Input: part model. Units: mm. Frame: model coordinates. A direction names the side the tool comes from. Coordinates: 2 decimals unless noted, no trailing zeros. Write each loop counter-clockwise with the first axis right and the second up, starting at its lowest first coordinate (ties: lowest second). Pieces come first, ordered by that corner, then holes.
1) Line query: L1, parallel to Y at x = 23.5, z = 0.7; L2, parallel to X at y = 24.5, z = 0.25; L3, parallel to Z at x = 19, y = 19.5. Output: solid intervals per line, ascending.
2) Draft query along Y for faces 3 (the flat face through (6, 6, -1.2)), 4 (the cylindrical face through (7.4, 32.5, 0.6)). Return one class per face: pulls with the +Y half, pulls with the -Y half, needs draft (parallel to the pull), parting line crosses it, or undercut.
3) Section query C-C (y = 103.5). Output: boundary loops of the cut face in (x, z).
4) Section query D-D (x = 6). Output: boundary loops of the cut face in (y, z).
5) Section query B-B (x = 18.5). Output: boundary loops of the cut face in (y, z).
6) Section query A-A (z = -0.6). Output: boundary loops of the cut face in (x, y), then the cut area to 3 significant figures.
7) Pin query (flat end, axial travel): pin 1 Ø0.6 at (x, z) = (6, -0.5) entering from -Y; pin 2 Ø0.6 at (y, z) = (104.5, -1) entering from -X; pin 3 Ø0.6 at (x, z) = (33.5, -0.5) entering from +Y. Return the tip coordinate at first contact, or that it passes through.
8) Set-up query: faces 1 (the flat face through (17, 56, 1.2)), 2 (the cylindrical face through (7.6, 77.5, 0.6)). Return all of +Z, -Z, +X, -X, +Y, -Y with unobstructed straight access to the full face (end or side cutting, diameter ignored); none if empty.
Autodesk Inventor part; units mm, degrees
ref_plane "YZ Plane" through (0, 0, 0) normal (1, 0, 0) x (0, 1, 0)
ref_plane "XZ Plane" through (0, 0, 0) normal (0, 1, 0) x (-1, 0, 0)
ref_plane "XY Plane" through (0, 0, 0) normal (0, 0, 1) x (1, 0, 0)
sketch "Skizze1" plane through (0, 0, 0) normal (0, 0, 1) x (1, 0, 0)
  line L0 (0, 0) -> (35, 0)
  line L1 (35, 0) -> (35, 110)
  line L2 (35, 110) -> (0, 110)
  line L3 (0, 110) -> (0, 0)
  line L4 (14, 105) -> (24, 105)
  line L5 (24, 105) -> (24, 100) construction
  line L6 (24, 100) -> (14, 100)
  line L7 (14, 100) -> (14, 105) construction
  line L8 (14, 10) -> (24, 10)
  line L9 (24, 10) -> (24, 5) construction
  line L10 (24, 5) -> (14, 5)
  line L11 (14, 5) -> (14, 10) construction
  line L12 (5, 90) -> (10, 90) construction
  line L13 (10, 90) -> (10, 80)
  line L14 (10, 80) -> (5, 80) construction
  line L15 (5, 80) -> (5, 90)
  line L16 (5, 30) -> (10, 30) construction
  line L17 (10, 30) -> (10, 20)
  line L18 (10, 20) -> (5, 20) construction
  line L19 (5, 20) -> (5, 30)
  line L20 (28, 90) -> (33, 90) construction
  line L21 (33, 90) -> (33, 80)
  line L22 (33, 80) -> (28, 80) construction
  line L23 (28, 80) -> (28, 90)
  line L24 (28, 30) -> (33, 30) construction
  line L25 (33, 30) -> (33, 20)
  line L26 (33, 20) -> (28, 20) construction
  line L27 (28, 20) -> (28, 30)
  line L28 (10, 80) -> (10, 30) construction
  line L29 (0, 55) -> (35, 55) construction
  arc A0 (5, 80) -> (10, 80) centre (7.5, 80) ccw
  arc A1 (10, 90) -> (5, 90) centre (7.5, 90) ccw
  arc A2 (33, 90) -> (28, 90) centre (30.5, 90) ccw
  arc A3 (28, 80) -> (33, 80) centre (30.5, 80) ccw
  arc A4 (24, 5) -> (24, 10) centre (24, 7.5) ccw
  arc A5 (14, 10) -> (14, 5) centre (14, 7.5) ccw
  arc A6 (5, 20) -> (10, 20) centre (7.5, 20) ccw
  arc A7 (28, 20) -> (33, 20) centre (30.5, 20) ccw
  arc A8 (33, 30) -> (28, 30) centre (30.5, 30) ccw
  arc A9 (10, 30) -> (5, 30) centre (7.5, 30) ccw
  arc A10 (24, 100) -> (24, 105) centre (24, 102.5) ccw
  arc A11 (14, 105) -> (14, 100) centre (14, 102.5) ccw
  line L30 (19, 10) -> (19, 100) construction
  line L31 (10, 85) -> (28, 85) construction
  point P0 (10, 55)
  point P1 (19, 85)
  dimension "d0" = 35
  dimension "d1" = 110
  dimension "d4" = 10
  dimension "d5" = 10
  dimension "d6" = 10
  dimension "d7" = 5
  dimension "d8" = 5
  dimension "d9" = 5
  dimension "d10" = 5
  dimension "d11" = 5
  dimension "d12" = 2
  dimension "d13" = 5
  dimension "d14" = 50
  dimension "d15" = 5
extrude "Extrusion2" add sketch "Skizze1" along normal blind 1.2
sketch "Skizze2" plane through (0, 0, 0) normal (0, 0, -1) x (-1, 0, 0)
  arc A0 (-28, 30) -> (-33, 30) centre (-30.5, 30) ccw construction
  line L0 (-28, 30) -> (-28, 20) construction
  arc A1 (-33, 20) -> (-28, 20) centre (-30.5, 20) ccw construction
  line L1 (-33, 20) -> (-33, 30) construction
  arc A2 (-28, 90) -> (-33, 90) centre (-30.5, 90) ccw construction
  line L2 (-28, 90) -> (-28, 80) construction
  arc A3 (-33, 80) -> (-28, 80) centre (-30.5, 80) ccw construction
  line L3 (-33, 80) -> (-33, 90) construction
  arc A4 (-5, 30) -> (-10, 30) centre (-7.5, 30) ccw construction
  line L4 (-5, 30) -> (-5, 20) construction
  arc A5 (-10, 20) -> (-5, 20) centre (-7.5, 20) ccw construction
  line L5 (-10, 20) -> (-10, 30) construction
  arc A6 (-5, 90) -> (-10, 90) centre (-7.5, 90) ccw construction
  line L6 (-5, 90) -> (-5, 80) construction
  arc A7 (-10, 80) -> (-5, 80) centre (-7.5, 80) ccw construction
  line L7 (-10, 80) -> (-10, 90) construction
  arc A8 (-24, 10) -> (-24, 5) centre (-24, 7.5) ccw construction
  line L8 (-24, 10) -> (-14, 10) construction
  arc A9 (-14, 5) -> (-14, 10) centre (-14, 7.5) ccw construction
  line L9 (-14, 5) -> (-24, 5) construction
  arc A10 (-24, 105) -> (-24, 100) centre (-24, 102.5) ccw construction
  line L10 (-24, 105) -> (-14, 105) construction
  arc A11 (-14, 100) -> (-14, 105) centre (-14, 102.5) ccw construction
  line L11 (-14, 100) -> (-24, 100) construction
  line L12 (0, 0) -> (-35, 0) construction
  line L13 (0, 110) -> (0, 0) construction
  line L14 (-35, 110) -> (0, 110) construction
  line L15 (-35, 0) -> (-35, 110) construction
  line L16 (-35, 3) -> (-30, 3)
  line L17 (-30, 3) -> (-30, 8)
  line L18 (-30, 8) -> (-35, 8)
  line L19 (-35, 8) -> (-35, 3)
  line L20 (-3, 3) -> (-8, 3)
  line L21 (-8, 3) -> (-8, 8)
  line L22 (-8, 8) -> (-3, 8)
  line L23 (-3, 8) -> (-3, 3)
  line L24 (-3, 102) -> (-8, 102)
  line L25 (-8, 102) -> (-8, 107)
  line L26 (-8, 107) -> (-3, 107)
  line L27 (-3, 107) -> (-3, 102)
  line L28 (-30, 107) -> (-35, 107)
  line L29 (-35, 107) -> (-35, 102)
  line L30 (-35, 102) -> (-30, 102)
  line L31 (-30, 102) -> (-30, 107)
  dimension "d18" = 5
  dimension "d19" = 5
  dimension "d20" = 5
  dimension "d21" = 5
  dimension "d22" = 3
  dimension "d23" = 0
  dimension "d24" = 3
  dimension "d25" = 3
extrude "Extrusion3" add sketch "Skizze2" along normal blind 1.2
properties part number "bett_V3_teil2_deckplatte_real" material "Holz (Walnuss)"
Answer:
1. L1: y = 0 to 5, 10 to 100, 105 to 110
1. L2: x = 0 to 5, 10 to 28, 33 to 35
1. L3: z = 0 to 1.2
2. face 3: needs draft
2. face 4: undercut
3. outline: (0, 0) - (3, 0) - (3, -1.2) - (8, -1.2) - (8, 0) - (11.71, 0) - (11.71, 1.2) - (0, 1.2) - close; (26.29, 0) - (30, 0) - (30, -1.2) - (35, -1.2) - (35, 1.2) - (26.29, 1.2) - close
4. outline: (0, 0) - (3, 0) - (3, -1.2) - (8, -1.2) - (8, 0) - (18, 0) - (18, 1.2) - (0, 1.2) - close; (32, 0) - (78, 0) - (78, 1.2) - (32, 1.2) - close; (92, 0) - (102, 0) - (102, -1.2) - (107, -1.2) - (107, 0) - (110, 0) - (110, 1.2) - (92, 1.2) - close
5. outline: (0, 0) - (5, 0) - (5, 1.2) - (0, 1.2) - close; (10, 0) - (100, 0) - (100, 1.2) - (10, 1.2) - close; (105, 0) - (110, 0) - (110, 1.2) - (105, 1.2) - close
6. outline: (3, 3) - (8, 3) - (8, 8) - (3, 8) - close; (3, 102) - (8, 102) - (8, 107) - (3, 107) - close; (30, 3) - (35, 3) - (35, 8) - (30, 8) - close; (30, 102) - (35, 102) - (35, 107) - (30, 107) - close
6. area: 100 mm2
7. pin 1: stops at y = 3
7. pin 2: stops at x = 3
7. pin 3: stops at y = 107
8. face 1: +Z, +X, -X, +Y, -Y
8. face 2: +Z, -Z
